Input: part model. Units: mm. Frame: model coordinates. Round coordinates to 2 decimals unless told otherwise and drop trailing zeros. Write each loop counter-clockwise with the first axis right and the second up, starting at its lowest first coordinate (ties: lowest second). Pieces come first, ordered by that corner, then holes. Notation, with made-up numbers: (73, 15.5) -> (77, 15.5) arc R21 ccw to (77, 23.5) -> close; hole circle Ø11 at (-8.75, -27). An arc over 180 degrees is marked (long way). Use CSV: the item, a comma, the result in double quotes.
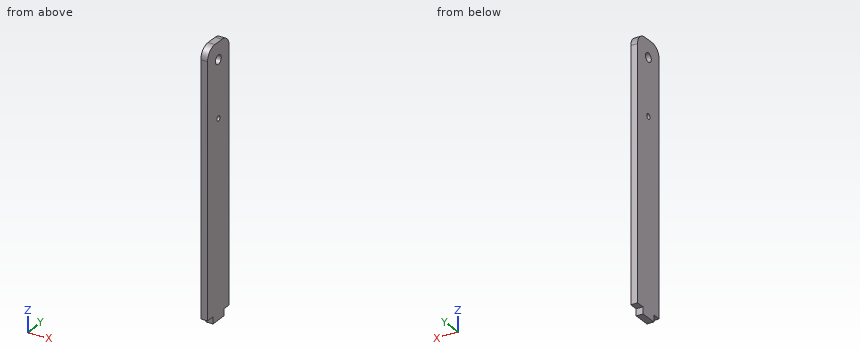
```python
from build123d import *

# Parameters (mm, degrees)
CROQUIS2_W                   = 230
CROQUIS2_H                   = 30
CROQUIS2_R                   = 4
SALIENTE_EXTRUIR1_DEPTH      = 3
TALADRO_DE_MARGEN_PARA_M41_D = 4.5
REDONDEO1_R                  = 10
CROQUIS5_W                   = 6
CROQUIS5_H                   = 15
SALIENTE_EXTRUIR2_DEPTH      = 6


with BuildPart() as part:
    # Croquis2 → Saliente-Extruir1 (new, symmetric)
    with BuildSketch(Plane(origin=(0, 0, 0), x_dir=(0, 0, -1), z_dir=(1, 0, 0))):
        Rectangle(CROQUIS2_W, CROQUIS2_H)
        with Locations((-100, 0)):
            Circle(CROQUIS2_R, mode=Mode.SUBTRACT)
    extrude(amount=SALIENTE_EXTRUIR1_DEPTH, both=True)

    # Taladro de margen para M41 (through all)
    with Locations(Plane(origin=(3, 0, 0), x_dir=(0, 0, -1), z_dir=(1, 0, 0))):
        with Locations((-50, 0)):
            Hole(TALADRO_DE_MARGEN_PARA_M41_D / 2)

    # Redondeo1
    redondeo1_edges = [part.edges().sort_by_distance(p)[0] for p in [
        (0, 15, 115),
        (0, -15, 115),
    ]]
    fillet(redondeo1_edges, radius=REDONDEO1_R)

    # Croquis5 → Saliente-Extruir2 (add, through all)
    with BuildSketch(Plane(origin=(3, 0, 0), x_dir=(0, 0, -1), z_dir=(1, 0, 0))):
        with Locations((118, 0)):
            Rectangle(CROQUIS5_W, CROQUIS5_H)
    extrude(amount=-SALIENTE_EXTRUIR2_DEPTH)


solid = part.part
```
Item 1: Section query C-C on x = 0.4. Return the cut outline in (y, z), plus the area to 3 significant figures.
Worked answers:
outline,"(-15, -115) -> (-7.5, -115) -> (-7.5, -121) -> (7.5, -121) -> (7.5, -115) -> (15, -115) -> (15, 105) arc R10 ccw to (5, 115) -> (-5, 115) arc R10 ccw to (-15, 105) -> close; hole circle Ø8 at (0, 100); hole circle Ø4.5 at (0, 50)"
area,"6,880 mm²"
Item 2: Section query B-B on y = 0. Return the cut outline in (x, z), plus the area to 3 significant figures.
Worked answers:
outline,"(-3, -121) -> (3, -121) -> (3, 47.75) -> (-3, 47.75) -> close; (-3, 52.25) -> (3, 52.25) -> (3, 96) -> (-3, 96) -> close; (-3, 104) -> (3, 104) -> (3, 115) -> (-3, 115) -> close"
area,"1,340 mm²"
Item 3: Section query A-A on z = 50. Return the cut outline in (x, y).
Worked answers:
outline,"(-3, -15) -> (3, -15) -> (3, -2.25) -> (-3, -2.25) -> close; (-3, 2.25) -> (3, 2.25) -> (3, 15) -> (-3, 15) -> close"
Item 4: First-contact query: pin 1 Ø13 at (y, z) = (0, 100) entering from -X. Flat tip, straight axial feed; report the tip coordinate or a pass-through.
Worked answers:
pin 1,"stops at x = -3"
Item 5: Section query D-D on z = 100. Return the cut outline in (x, y), plus the area to 3 significant figures.
Worked answers:
outline,"(-3, -15) -> (3, -15) -> (3, -4) -> (-3, -4) -> close; (-3, 4) -> (3, 4) -> (3, 15) -> (-3, 15) -> close"
area,"132 mm²"
Item 6: Line query: line 1 (Y direction, x = 1.45, z = 50); line 2 (Y direction, x = 1.35, z = 100); line 3 (Z direction, x = 0.3, y = 2). Output: solid intervals per line, ascending.
Worked answers:
line 1,"y = -15 to -2.25, 2.25 to 15"
line 2,"y = -15 to -4, 4 to 15"
line 3,"z = -121 to 48.97, 51.03 to 96.54, 103.46 to 115"
